```python
from build123d import *

# Parameters (mm, degrees)
BOSS_EXTRU_1_DEPTH      = 1.5
ESQUISSE4_R             = 4
ESQUISSE4_R_2           = 1.5
ESQUISSE4_W             = 168
ESQUISSE4_H             = 102
ENL_V_MAT_EXTRU_3_DEPTH = 3
ENL_V_MAT_EXTRU_4_DEPTH = 1.5
ESQUISSE11_R            = 1.5
ENL_V_MAT_EXTRU_5_DEPTH = 1.5
CONG_1_R                = 1
ESQUISSE12_R            = 1.5
ENL_V_MAT_EXTRU_6_DEPTH = 224.924001117
ESQUISSE14_W            = 27
ESQUISSE14_H            = 11
ENL_V_MAT_EXTRU_7_DEPTH = 1.5
CONG_2_R                = 1.5


# Read off the part's stored shape, not the designer's step: Enlèv. mat.-Extru.4
with BuildPart() as part:
    # Esquisse1 → Boss.-Extru.1 (new body)
    with BuildSketch(Plane(origin=(0, 0, 0), x_dir=(1, 0, 0), z_dir=(0, 1, 0))):
        with BuildLine():
            Line((-165, 6.391802297), (-165, 0))
            Line((-165, 0), (165, 0))
            Line((165, 0), (165, 6.391802297))
            add(Edge.make_bspline(
                [(165, 6.391802297), (0, 608.094924715), (-165, 6.391802297)],
                knots=[1.893832827, 1.893832827, 1.893832827, 4.38935248, 4.38935248, 4.38935248], degree=2, weights=[1, 0.317447459, 1]))
        make_face()
    extrude(amount=BOSS_EXTRU_1_DEPTH)

    # Esquisse4 → Enlèv. mat.-Extru.3 (cut)
    with BuildSketch(Plane(origin=(0, 1.5, 0), x_dir=(1, 0, 0), z_dir=(0, 1, 0))):
        with Locations(Location((-117.74, 61, 0), (0, 0, 270))):
            Circle(ESQUISSE4_R)
        with Locations(Location((-112.919092927, 55.254666677, 0), (0, 0, 270))):
            Circle(ESQUISSE4_R_2)
        with Locations(Location((-122.560907073, 66.745333323, 0), (0, 0, 270))):
            Circle(ESQUISSE4_R_2)
        with Locations(Location((-101.74, 61, 0), (0, 0, 270))):
            Circle(ESQUISSE4_R_2)
        with Locations(Location((104.26, 61, 0), (0, 0, 270))):
            Circle(ESQUISSE4_R_2)
        with Locations((1.26, 59)):
            Rectangle(ESQUISSE4_W, ESQUISSE4_H)
    extrude(amount=-ENL_V_MAT_EXTRU_3_DEPTH, mode=Mode.SUBTRACT)

    # Enlèv. mat.-Extru.4 outline → Enlèv. mat.-Extru.4 (cut)
    with BuildSketch(Plane(origin=(0, 0, 0), x_dir=(1, 0, 0), z_dir=(0, 1, 0))):
        with BuildLine():
            add(Edge.make_bspline(
                [(131.492595534, 29.994209065), (131.937846155, 45.779047079), (119, 45.779047079), (106.062153845, 45.779047079), (106.507404466, 29.994209065)],
                knots=[1.536374944, 1.536374944, 1.536374944, 3.141592654, 3.141592654, 4.746810363, 4.746810363, 4.746810363], degree=2, weights=[1, 0.694832863, 1, 0.694832863, 1]))
            add(Edge.make_bspline(
                [(106.507404466, 29.994209065), (106.062153845, 14.209371052), (119, 14.209371052), (131.937846155, 14.209371052), (131.492595534, 29.994209065)],
                knots=[4.677967597, 4.677967597, 4.677967597, 6.283185307, 6.283185307, 7.888403017, 7.888403017, 7.888403017], degree=2, weights=[1, 0.694832863, 1, 0.694832863, 1]))
        make_face()
    extrude(amount=ENL_V_MAT_EXTRU_4_DEPTH, mode=Mode.SUBTRACT)

    # Esquisse11 → Enlèv. mat.-Extru.5 (cut)
    with BuildSketch(Plane(origin=(0, 1.5, 0), x_dir=(1, 0, 0), z_dir=(0, 1, 0))):
        with Locations(Location((103, 29.994209065, 0), (0, 0, 270))):
            Circle(ESQUISSE11_R)
        with Locations(Location((135, 29.994209065, 0), (0, 0, 90))):
            Circle(ESQUISSE11_R)
    extrude(amount=-ENL_V_MAT_EXTRU_5_DEPTH, mode=Mode.SUBTRACT)

    # Congé1
    cong_1_edges = [part.edges().sort_by_distance(p)[0] for p in [
        (-82.74, 0.75, -110),
        (-82.74, 0.75, -8),
        (85.26, 0.75, -8),
        (85.26, 0.75, -110),
        (165, 0.75, 0),
        (-165, 0.75, 0),
    ]]
    fillet(cong_1_edges, radius=CONG_1_R)

    # Esquisse12 → Enlèv. mat.-Extru.6 (cut, through all)
    with BuildSketch(Plane(origin=(0, 1.5, 0), x_dir=(1, 0, 0), z_dir=(0, 1, 0))):
        with Locations(Location((-156, 15, 0), (0, 0, 270))):
            Circle(ESQUISSE12_R)
        with Locations(Location((-76, 123, 0), (0, 0, 270))):
            Circle(ESQUISSE12_R)
        with Locations(Location((-25, 143, 0), (0, 0, 270))):
            Circle(ESQUISSE12_R)
        with Locations(Location((25, 143, 0), (0, 0, 270))):
            Circle(ESQUISSE12_R)
        with Locations(Location((76, 123, 0), (0, 0, 270))):
            Circle(ESQUISSE12_R)
        with Locations(Location((156, 15, 0), (0, 0, 270))):
            Circle(ESQUISSE12_R)
        with Locations(Location((-102, 6, 0), (0, 0, 270))):
            Circle(ESQUISSE12_R)
        with Locations(Location((102, 6, 0), (0, 0, 270))):
            Circle(ESQUISSE12_R)
        with Locations(Location((-118, 86, 0), (0, 0, 270))):
            Circle(ESQUISSE12_R)
        with Locations(Location((118, 86, 0), (0, 0, 270))):
            Circle(ESQUISSE12_R)
        with BuildLine():
            Line((-4, 0), (4, 0))
            ThreePointArc((4, 0), (0, 2.438447187), (-4, 0))
        make_face()
    extrude(amount=-ENL_V_MAT_EXTRU_6_DEPTH, mode=Mode.SUBTRACT)

    # Esquisse14 → Enlèv. mat.-Extru.7 (cut)
    with BuildSketch(Plane(origin=(0, 1.5, 0), x_dir=(1, 0, 0), z_dir=(0, 1, 0))):
        with Locations((0, 131)):
            Rectangle(ESQUISSE14_W, ESQUISSE14_H)
    extrude(amount=-ENL_V_MAT_EXTRU_7_DEPTH, mode=Mode.SUBTRACT)

    # Congé2
    cong_2_edges = [part.edges().sort_by_distance(p)[0] for p in [
        (-13.5, 0.75, -125.5),
        (-13.5, 0.75, -136.5),
        (13.5, 0.75, -136.5),
        (13.5, 0.75, -125.5),
    ]]
    fillet(cong_2_edges, radius=CONG_2_R)


solid = part.part
```
Design review of the part built by this model. Coordinates are the model's own, in mm. Give positions to 0.01 mm unless a question says otherwise; leave off trailing zeros. Write each question's results on one line, items separated by ' | '.
Q1. Wall thickness on L1, parallel to X at y = 0.55, z = -6; L2, parallel to X at y = 0.8, z = -86; L3, parallel to X at y = 0.5, z = -61: over which ranges is each line inside the solid? List them lowest first.
Reply:
L1: x = -165 to -103.5, -100.5 to 100.5, 103.5 to 165 | L2: x = -125.57 to -119.5, -116.5 to -82.74, 85.26 to 116.5, 119.5 to 125.57 | L3: x = -142.42 to -121.74, -113.74 to -103.24, -100.24 to -82.74, 85.26 to 102.76, 105.76 to 142.42
Q2. The part is to be moulded in two halves that separate along Z. For faces 1 (the face through (-114.4, 0.8, -58.8)), 2 (the face through (-13, 1.5, -125)), say which applies: +Z half, -Z half, draft (parallel to the pull), parting line (faces both ways), or undercut.
Reply:
face 1: undercut | face 2: draft
Q3. For pin 1 Ø0.8 at (x, y) = (19.5, 0.5) entering from -Z; pin 2 Ø0.8 at (y, z) = (1, -59.5) entering from -X, all flat-tipped, find the tip position at first contact; note any pin that passes through.
Reply:
pin 1: stops at z = -150.09 | pin 2: stops at x = -143.5
Q4. Take a section at A-A, the plane y = 0.9. Give the number of separate pieces and of enclosed holes in the cut face, plus the area to 3 significant figures.
Reply:
separate pieces: 1 | enclosed holes: 20 | area: 18,900 mm²
